```python
from build123d import *

# Parameters (mm, degrees)
F1_START      = -7
F0_R          = 2.45
F0_R_2        = 3.2
F0_R_3        = 15
F1_DEPTH      = 5
F3_DEPTH      = 40
F3_DEPTH_BACK = 40


with BuildPart() as f1:
    # F0 (on Top) → F1 (new body)
    with BuildSketch(Plane.XY.offset(F1_START)):
        with BuildLine():
            Line((48.9758001545, -7.5026887111), (50.3920186759, -7.0373422574))
            ThreePointArc((50.3920186759, -7.0373422574), (47.6313972081, 42.5), (6.1111111111, 69.65943945))
            Line((6.1111111111, 69.65943945), (5, 68.66563146))
            Line((5, 68.66563146), (5, 65))
            ThreePointArc((5, 65), (0, 60), (-5, 65))
            Line((-5, 65), (-5, 68.66563146))
            Line((-5, 68.66563146), (-6.1111111111, 69.65943945))
            ThreePointArc((-6.1111111111, 69.65943945), (-47.3563637716, 42.9709637004), (-50.8191344463, -6.0336771423))
            ThreePointArc((-50.8191344463, -6.0336771423), (-50.6080647229, -6.5365685522), (-50.3920186759, -7.0373422574))
            Line((-50.3920186759, -7.0373422574), (-48.9758001545, -7.5026887111))
            Line((-48.9758001545, -7.5026887111), (-45.8012701892, -5.6698729811))
            ThreePointArc((-45.8012701892, -5.6698729811), (-38.9711431703, -7.5), (-40.8012701892, -14.3301270189))
            Line((-40.8012701892, -14.3301270189), (-43.9758001545, -16.1629427489))
            Line((-43.9758001545, -16.1629427489), (-44.2809075648, -17.6220971926))
            ThreePointArc((-44.2809075648, -17.6220971926), (0, -40), (44.2809075648, -17.6220971926))
            Line((44.2809075648, -17.6220971926), (43.9758001545, -16.1629427489))
            Line((43.9758001545, -16.1629427489), (40.8012701892, -14.3301270189))
            ThreePointArc((40.8012701892, -14.3301270189), (38.9711431703, -7.5), (45.8012701892, -5.6698729811))
            Line((45.8012701892, -5.6698729811), (48.9758001545, -7.5026887111))
        make_face()
        with Locations((0, -32)):
            Circle(F0_R, mode=Mode.SUBTRACT)
        with Locations((-13, -24)):
            Circle(F0_R_2, mode=Mode.SUBTRACT)
        Circle(F0_R_3, mode=Mode.SUBTRACT)
        with Locations((13, -24)):
            Circle(F0_R_2, mode=Mode.SUBTRACT)
        with Locations((-13, 24)):
            Circle(F0_R_2, mode=Mode.SUBTRACT)
        with Locations((0, 32)):
            Circle(F0_R, mode=Mode.SUBTRACT)
        with Locations((13, 24)):
            Circle(F0_R_2, mode=Mode.SUBTRACT)
    extrude(amount=-F1_DEPTH)

    # F2 (on Top) → F3 (cut, two sides)
    with BuildSketch(Plane.XY) as f3_sk:
        with BuildLine():
            Line((0, -13), (-8, -13))
            ThreePointArc((-8, -13), (-10, -15), (-8, -17))
            Line((-8, -17), (0, -17))
            Line((0, -17), (8, -17))
            ThreePointArc((8, -17), (10, -15), (8, -13))
            Line((8, -13), (0, -13))
        make_face()
    extrude(amount=-F3_DEPTH, mode=Mode.SUBTRACT)
    extrude(f3_sk.sketch, amount=F3_DEPTH_BACK, mode=Mode.SUBTRACT)


solid = f1.part
```
For this review, take the finished solid that the model builds, in its own axes (mm). A direction names the side the tool comes from. Coordinates: 2 decimals unless noted, no trailing zeros. Order: outer loops, then holes, each group sorted by start corner. A loop starts at its lowest first (then second) coordinate and runs counter-clockwise, first axis right, second up. Notation, with made-up numbers: (-1, 62) -> (22, 62) arc R22 ccw to (22, 76) -> close; hole circle Ø1 at (66.5, 61). An arc over 180 degrees is marked (long way). Answer as CSV lines item,"result".
Q1. Clearance check with flat-ended pins moving along their axes: pin 1 Ø1.8 at (y, z) = (66, -8.5) entering from +X; pin 2 Ø1 at (x, z) = (12.5, -8.5) entering from -Y; pin 3 Ø0.6 at (x, z) = (-8, -10) entering from -Y. State where each tip first meets the part, or that it passes through.
Model answer:
pin 1,"stops at x = 22.69"
pin 2,"stops at y = -38.67"
pin 3,"stops at y = -39.46"
Q2. We need section C-C (y = -32). State the section outline as (x, z) points.
Model answer:
outline,"(-28.57, -12) -> (-2.45, -12) -> (-2.45, -7) -> (-28.57, -7) -> close; (2.45, -12) -> (28.57, -12) -> (28.57, -7) -> (2.45, -7) -> close"
Q3. Wall thickness on line 1 along Y through (x, z) = (0, -10); line 2 along X through (y, z) = (-23.5, -8.3); line 3 along Y through (x, z) = (-13, -9.1): over which ranges is each line inside the solid? List them lowest first. Write a range as [from, to].
Model answer:
line 1,"y = [-40, -34.45], [-29.55, -17], [15, 29.55], [34.45, 60]"
line 2,"x = [-39.28, -16.16], [-9.84, 9.84], [16.16, 39.28]"
line 3,"y = [-38.44, -27.2], [-20.8, -7.48], [7.48, 20.8], [27.2, 68.44]"
Q4. We need section B-B (z = -9.8). Count the separate pieces of the cut face and the enclosed holes in it, plus the area to 3 significant figures.
Model answer:
separate pieces,"1"
enclosed holes,"7"
area,"8,300 mm2"
Q5. For faces 1 (the face through (-10, -15, -9)), 2 (the face through (-1, 16, -12)), 3 (the face through (5, 67, -9)), 4 (the face through (42.41, -15.26, -9.46)), list the 3-axis set-ups (+Z, -Z, +X, -X, +Y, -Y) from which the entire face can be reached by the end or side of a thin tool; tool diameter is ignored.
Model answer:
face 1,"+Z, -Z"
face 2,"-Z, +X, -X, +Y, -Y"
face 3,"+Z, -Z, +Y"
face 4,"+Z, -Z, +X"
Q6. We need section A-A (x = 0). State the section outline as (y, z) points.
Model answer:
outline,"(-40, -12) -> (-34.45, -12) -> (-34.45, -7) -> (-40, -7) -> close; (-29.55, -12) -> (-17, -12) -> (-17, -7) -> (-29.55, -7) -> close; (15, -12) -> (29.55, -12) -> (29.55, -7) -> (15, -7) -> close; (34.45, -12) -> (60, -12) -> (60, -7) -> (34.45, -7) -> close"
Q7. Draft analysis for pull direction Y (two halves, no side actions). For faces 5 (the face through (0, 60, -9)), 6 (the face through (14.72, 26.7, -9.46)), 7 (the face through (-47.41, -6.6, -9.46)), state which applies: released by +Y, released by -Y, zero draft, split by the parting line, or undercut.
Model answer:
face 5,"released by +Y"
face 6,"undercut"
face 7,"released by -Y"
Q8. We need section D-D (x = 42.5). State the section outline as (y, z) points, plus the area to 3 significant figures.
Model answer:
outline,"(-19.91, -12) -> (-15.31, -12) -> (-15.31, -7) -> (-19.91, -7) -> close; (-5.06, -12) -> (49.91, -12) -> (49.91, -7) -> (-5.06, -7) -> close"
area,"298 mm2"
